Here's how the part is built. I have some questions about the finished solid (model axes, mm). Face numbers are marked on the shaded views. A direction names the side the tool comes from. Give positions to 0.01 mm unless a question says otherwise; leave off trailing zeros. Loops run counter-clockwise (first coordinate to the right, second up) from the corner with the lowest first, then second, coordinate; pieces in that order, holes last.
Q1. I need wall thicknesses on line 1 (Z direction, x = -10.5, y = 4.25) (3 decimals); line 2 (X direction, y = 10.5, z = -5); line 3 (Y direction, x = 9, z = 0) (3 decimals). Which ranges of each line are inside material? Lowest first, please.
Q2. If we section it at D-D (y = 6.5): Please give me the cut outline in (x, z) (3 decimals).
Q3. Will these pins go through, and if not, where does the flat tip stop? P1, Ø2.5, axis at x = -12.7, y = 9.525, coming from the +Z side; P2, Ø4, axis at x = 12.7, y = 9.525, coming from the -Z side; P3, Ø1.6, axis at y = 17, z = 0, coming from the -X side; P4, Ø1.6, axis at y = 20.32, z = 0, coming from the -X side.
Q4. For the marked faces 1 and 2, which set-ups out of +Z, -Z, +X, -X, +Y, -Y let a thin tool reach every point of the face, with its end or its side?
Q5. If we section it at C-C (x = 3.5): Please give me the cut outline in (y, z) (3 decimals), plus the area to 3 significant figures.
Q6. If we section it at A-A (z = 0): Please give me the cut outline in (x, y) (3 decimals), plus the area to 3 significant figures.
Q7. If we section it at B-B (z = -4.5): Give the number of separate pieces and of enclosed holes in the cut face, plus the area to 3 significant figures.
Q8. We'd pull the mould along Z, two halves only. Please class the marked faces 3, 4 and 5: +Z half, -Z half, draft (parallel to the pull), parting line (faces both ways), or undercut.
from build123d import *

# Parameters (mm, degrees)
SKETCH1_W           = 44.45
SKETCH1_H           = 19.05
BOSS_EXTRUDE1_DEPTH = 19.05
SKETCH2_R           = 1.5875
CUT_EXTRUDE1_DEPTH  = 19.05
SKETCH9_W           = 2.54
SKETCH9_H           = 5.08
BOSS_EXTRUDE2_DEPTH = 2.54
SKETCH3_R           = 0.508
SKETCH3_W           = 6.35
SKETCH3_H           = 12.7
CUT_EXTRUDE2_DEPTH  = 38.1
SKETCH4_W           = 16.467967332
SKETCH4_H           = 6.35
CUT_EXTRUDE3_DEPTH  = 43.18
CUT_EXTRUDE4_DEPTH  = 19.05
SKETCH7_W           = 15.04890267
SKETCH7_H           = 6.35
CUT_EXTRUDE5_DEPTH  = 3.81


with BuildPart() as part:
    # Sketch1 → Boss-Extrude1 (new body)
    with BuildSketch(Plane(origin=(0, 0, 0), x_dir=(1, 0, 0), z_dir=(0, 1, 0))):
        Rectangle(SKETCH1_W, SKETCH1_H)
    extrude(amount=BOSS_EXTRUDE1_DEPTH)

    # Sketch2 → Cut-Extrude1 (cut)
    with BuildSketch(Plane.XY.offset(9.525)):
        with Locations((-12.7, 9.525)):
            Circle(SKETCH2_R)
        with Locations((12.7, 9.525)):
            Circle(SKETCH2_R)
        with BuildLine():
            ThreePointArc((-12.7, 19.05), (-22.225, 9.525), (-12.7, 0))
            ThreePointArc((-12.7, 0), (-32.914765451, 9.525), (-12.7, 19.05))
        make_face()
        with BuildLine():
            ThreePointArc((12.7, 19.05), (32.914765451, 9.525), (12.7, 0))
            ThreePointArc((12.7, 0), (22.225, 9.525), (12.7, 19.05))
        make_face()
    extrude(amount=-CUT_EXTRUDE1_DEPTH, mode=Mode.SUBTRACT)

    # Sketch9 → Boss-Extrude2 (add)
    with BuildSketch(Plane(origin=(0, 19.05, 0), x_dir=(1, 0, 0), z_dir=(0, 1, 0))):
        with Locations((1.27, 0)):
            Rectangle(SKETCH9_W, SKETCH9_H)
    extrude(amount=BOSS_EXTRUDE2_DEPTH)

    # Sketch3 → Cut-Extrude2 (cut, symmetric)
    with BuildSketch(Plane(origin=(0, 0, 0), x_dir=(0, 0, -1), z_dir=(1, 0, 0))):
        with Locations((0, 20.32)):
            Circle(SKETCH3_R)
        with Locations((0, 9.525)):
            Rectangle(SKETCH3_W, SKETCH3_H)
        with BuildLine():
            ThreePointArc((-2.54, 19.05), (0, 21.59), (2.54, 19.05))
            ThreePointArc((2.54, 19.05), (0, 24.1080653), (-2.54, 19.05))
        make_face()
    extrude(amount=CUT_EXTRUDE2_DEPTH, both=True, mode=Mode.SUBTRACT)

    # Sketch4 → Cut-Extrude3 (cut)
    with BuildSketch(Plane(origin=(0, 19.05, 0), x_dir=(1, 0, 0), z_dir=(0, 1, 0))):
        Polygon((-29.361154188, -9.525), (-12.7, -9.525), (1.5875, -9.525), (28.406626571, -9.525), (28.406626571, -6.35), (1.5875, -6.35), (-12.7, -6.35), (-29.361154188, -6.35), align=None)
        Polygon((-12.7, 6.35), (-31.510324581, 6.35), (-31.510324581, 9.525), (-11.1125, 9.525), (1.5875, 9.525), (30.675017081, 9.525), (30.675017081, 6.35), (1.5875, 6.35), align=None)
        with Locations((20.933983666, 0)):
            Rectangle(SKETCH4_W, SKETCH4_H)
    extrude(amount=-CUT_EXTRUDE3_DEPTH, mode=Mode.SUBTRACT)

    # Sketch6 → Cut-Extrude4 (cut)
    with BuildSketch(Plane.XY.offset(9.525)):
        with BuildLine():
            Line((12.7, 0), (31.980086248, 0))
            Line((31.980086248, 0), (31.980086248, 3.175))
            Line((31.980086248, 3.175), (26.13215645, 13.808491056))
            Line((26.13215645, 13.808491056), (19.05, 19.755698555))
            Line((19.05, 19.755698555), (19.05, 9.525))
            ThreePointArc((19.05, 9.525), (17.190128061, 5.034871939), (12.7, 3.175))
            Line((12.7, 3.175), (12.7, 0))
        make_face()
        with BuildLine():
            Line((-12.7, 0), (-12.7, 3.175))
            ThreePointArc((-12.7, 3.175), (-17.190128061, 5.034871939), (-19.05, 9.525))
            Line((-19.05, 9.525), (-19.05, 20.942771878))
            Line((-19.05, 20.942771878), (-28.921644245, 11.767684684))
            Line((-28.921644245, 11.767684684), (-28.921644245, 0))
            Line((-28.921644245, 0), (-12.7, 0))
        make_face()
    extrude(amount=-CUT_EXTRUDE4_DEPTH, mode=Mode.SUBTRACT)

    # Sketch7 → Cut-Extrude5 (cut)
    with BuildSketch(Plane(origin=(0, 19.05, 0), x_dir=(1, 0, 0), z_dir=(0, 1, 0))):
        with Locations((-20.224451335, 0)):
            Rectangle(SKETCH7_W, SKETCH7_H)
    extrude(amount=-CUT_EXTRUDE5_DEPTH, mode=Mode.SUBTRACT)


solid = part.part
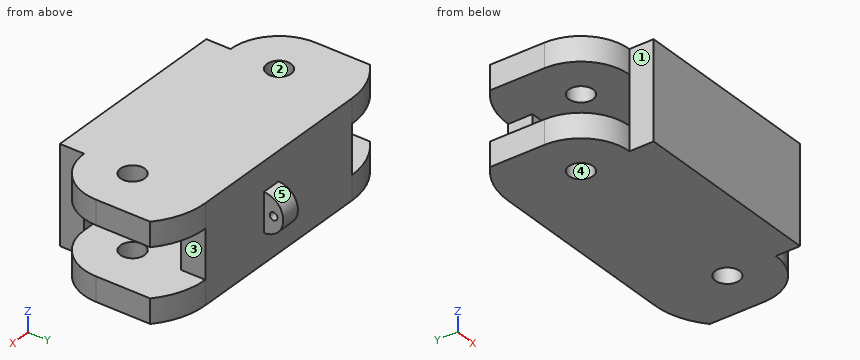
Check sheet entries:
1. line 1: z = -6.35 to -3.175, 3.175 to 6.35
1. line 2: x = -19.05 to -13.95, -11.45 to 11.45, 13.95 to 19.05
1. line 3: y = 0 to 3.175, 15.875 to 19.05
2. outline: (-18.283, -6.35) - (18.283, -6.35) - (18.283, -3.175) - (-18.283, -3.175) - close; (-18.283, 3.175) - (18.283, 3.175) - (18.283, 6.35) - (-18.283, 6.35) - close
3. P1: passes through
3. P2: stops at z = -6.35
3. P3: stops at x = -12.7
3. P4: stops at x = 0
4. face 1: +Z, -Z, -X, -Y
4. face 2: +Z, -Z
5. outline: (0, -6.35) - (19.05, -6.35) - (19.05, 6.35) - (0, 6.35) - close; hole (3.175, -3.175) - (15.875, -3.175) - (15.875, 3.175) - (3.175, 3.175) - close
5. area: 161 mm2
6. outline: (-12.7, 0) - (12.7, 0) - (12.7, 3.175) - (-12.7, 3.175) - close; (-12.7, 15.875) - (12.7, 15.875) - (12.7, 19.05) - (2.54, 19.05) - (2.54, 19.812) - (0, 19.812) - (0, 19.05) - (-12.7, 19.05) - close; (0, 20.828) - (2.54, 20.828) - (2.54, 21.59) - (0, 21.59) - close
6. area: 165 mm2
7. separate pieces: 1
7. enclosed holes: 2
7. area: 643 mm2
8. face 3: undercut
8. face 4: draft
8. face 5: parting line
